Source: CAD feature listing. Evaluate the final solid. Frame: model axes, mm. A direction names the side the tool comes from. Give positions to 0.01 mm unless a question says otherwise; leave off trailing zeros. Loops run counter-clockwise (first coordinate to the right, second up) from the corner with the lowest first, then second, coordinate; pieces in that order, holes last. Notation, with made-up numbers: (47, -18.5) -> (60, -18.5) arc R28 ccw to (60, 9.5) -> close; hole circle Ø5 at (54, 53.5). An arc over 180 degrees is marked (long way). Return JSON: item names as keys, results as strings. Group by question number.
(1) Cut plane C-C on z = 40. Return loops of the section in (x, y), then the cut area to 3 significant figures.
(2) Draft query along Z for faces 4 (the face through (13.195, 2.028, 85.487)), 5 (the face through (13, 2, 124)), 6 (the face through (0, 3, 54)), 7 (the face through (13, 5, -5)). Return one class per face: released by +Z, released by -Z, zero draft, split by the parting line, or undercut.
(3) Ray query, line 1 (Z direction, x = 13, y = 3.05); line 2 (X direction, y = 3.75, z = 104); line 3 (Z direction, x = 1.5, y = 4.5). Return the intervals inside material, ascending. Write a range as from..to.
(4) Cut plane A-A on x = 13. Return loops of the section in (y, z), then the cut area to 3 significant figures.
(5) Cut plane B-B on y = 8. Return loops of the section in (x, z), then the cut area to 3 significant figures.
(6) Access query for faces 1 (the face through (13, 0, 59)), 2 (the face through (2, 4, 61)), 3 (the face through (4.5, 3, 63)). Directions: +Z, -Z, +X, -X, +Y, -Y. A direction counts if a zero-diameter tool reaches every point of the face in a straight line with its end or side. Return the directions, or none.
(7) Cut plane D-D on z = 92. Return loops of the section in (x, y), then the cut area to 3 significant figures.
(8) Pin query (flat end, axial travel): pin 1 (1.5 mm diameter, centred on x = 7.5, y = 6.5, fed in from +Z); pin 2 (12 mm diameter, centred on x = 8, z = 10.5, fed in from +Y); pin 3 (0.6 mm diameter, centred on x = 20.5, z = 35, fed in from +Y). Return the tip coordinate at first contact, or that it passes through.
Autodesk Fusion 360 part; units mm, degrees
sketch "Eskiz1" plane through (0, 0, 0) normal (0, 1, 0) x (1, 0, 0)
  line L0 (0, 0) -> (26, 0)
  line L1 (26, 0) -> (26, -124)
  line L2 (26, -124) -> (0, -124)
  line L3 (0, -124) -> (0, 0)
  line L4 (4.5, 0) -> (6.5, 0)
  line L5 (6.5, 0) -> (6.5, -124)
  line L6 (6.5, -124) -> (4.5, -124)
  line L7 (4.5, -124) -> (4.5, 0)
  line L8 (19.5, 0) -> (21.5, 0)
  line L9 (21.5, 0) -> (21.5, -124)
  line L10 (21.5, -124) -> (19.5, -124)
  line L11 (19.5, -124) -> (19.5, 0)
  line L12 (0, 0) -> (26, 0)
  line L13 (26, 0) -> (26, 5)
  line L14 (26, 5) -> (0, 5)
  line L15 (0, 5) -> (0, 0)
  line L16 (0, -124) -> (26, -124)
  line L17 (26, -124) -> (26, -129)
  line L18 (26, -129) -> (0, -129)
  line L19 (0, -129) -> (0, -124)
  dimension "d1" = 26
  dimension "d2" = 124
  dimension "d3" = 2
  dimension "d4" = 4.5
  dimension "d5" = 2
  dimension "d6" = 13
  dimension "d11" = 5
  dimension "d18" = 5
extrude "Ekstrüde Et1" add sketch "Eskiz1" along normal blind 2 contours L0 L2 L4 L5 L6 L7 L12 L16 | L0 L2 L8 L9 L10 L11 L12 L16 makes body 1 at (6.5, 0.6667, 41.3333) makes body 2 at (21.5, 0.6667, 41.3333)
extrude "Ekstrüde Et2" add sketch "Eskiz1" along normal blind 4 contours L0 L2 L3 L7 L12 L16 | L0 L2 L5 L11 L12 L16 | L0 L1 L2 L9 L12 L16 bodies 1 2
extrude "Ekstrüde Et3" add sketch "Eskiz1" along normal blind 12 contours L0 L4 L8 L12 L13 L14 L15 bodies 1
sketch "Eskiz2" plane through (0, 0, -5) normal (0, 0, -1) x (-1, 0, 0)
  line L0 (-26, 0) -> (0, 0)
  line L1 (0, 0) -> (0, 12)
  line L2 (0, 12) -> (-26, 12)
  line L3 (-26, 12) -> (-26, 0)
  circle A0 centre (-13, 8) radius 2.5
  dimension "d14" = 5
  dimension "d15" = 4
extrude "Ekstrüde Et4" cut sketch "Eskiz2" against normal blind 6 contours A0 bodies 1
sketch "Eskiz3" plane through (0, 4, 0) normal (0, 1, 0) x (-1, 0, 0)
  line L0 (-6.5, 0) -> (-6.5, 124)
  line L1 (-6.5, 124) -> (-19.5, 124)
  line L2 (-19.5, 124) -> (-19.5, 0)
  line L3 (-19.5, 0) -> (-6.5, 0)
  circle A0 centre (-13, 84) radius 1.5
  circle A1 centre (-13, 40) radius 1.5
  dimension "d19" = 3
  dimension "d20" = 3
  dimension "d21" = 40
  dimension "d22" = 40
extrude "Ekstrüde Et5" cut sketch "Eskiz3" against normal blind 15 contours A0 | A1 bodies 1
Answers:
{
 "1": {"outline": "(0, 0) -> (11.5, 0) -> (11.5, 4) -> (6.5, 4) -> (6.5, 2) -> (4.5, 2) -> (4.5, 4) -> (0, 4) -> close; (14.5, 0) -> (26, 0) -> (26, 4) -> (21.5, 4) -> (21.5, 2) -> (19.5, 2) -> (19.5, 4) -> (14.5, 4) -> close", "area": "84.0 mm²"},
 "2": {"face 4": "undercut", "face 5": "released by +Z", "face 6": "zero draft", "face 7": "released by -Z"},
 "3": {"line 1": "-5..38.5, 41.5..82.5, 85.5..124", "line 2": "0..4.5, 6.5..19.5, 21.5..26", "line 3": "-5..0"},
 "4": {"outline": "(0, -5) -> (5.5, -5) -> (5.5, 0) -> (4, 0) -> (4, 38.5) -> (0, 38.5) -> close; (0, 41.5) -> (4, 41.5) -> (4, 82.5) -> (0, 82.5) -> close; (0, 85.5) -> (4, 85.5) -> (4, 124) -> (0, 124) -> close; (10.5, -5) -> (12, -5) -> (12, 0) -> (10.5, 0) -> close", "area": "507 mm²"},
 "5": {"outline": "(0, -5) -> (10.5, -5) -> (10.5, 0) -> (0, 0) -> close; (15.5, -5) -> (26, -5) -> (26, 0) -> (15.5, 0) -> close", "area": "105 mm²"},
 "6": {"face 1": "+Z, -Z, +X, -X, -Y", "face 2": "+Z, +X, -X, +Y", "face 3": "+Z, +Y"},
 "7": {"outline": "(0, 0) -> (26, 0) -> (26, 4) -> (21.5, 4) -> (21.5, 2) -> (19.5, 2) -> (19.5, 4) -> (6.5, 4) -> (6.5, 2) -> (4.5, 2) -> (4.5, 4) -> (0, 4) -> close", "area": "96.0 mm²"},
 "8": {"pin 1": "z = 0", "pin 2": "y = 4", "pin 3": "y = 2"}
}
